Source: CAD feature listing. Evaluate the final solid. Frame: model axes, mm. Give positions to 0.01 mm unless a question says otherwise; leave off trailing zeros.
from build123d import *

# Parameters (mm, degrees)
SKETCH_1_R          = 3.2
SKETCH_1_R_2        = 2.5
EXTRUDE_1_DEPTH     = 3
SKETCH_2_R          = 2
SKETCH_2_R_2        = 1.75
CUT_EXTRUDE_1_DEPTH = 10


with BuildPart() as part:
    # Эскиз1 → Бобышка-Вытянуть1 (new body)
    with BuildSketch(Plane(origin=(0, 0, 0), x_dir=(1, 0, 0), z_dir=(0, 1, 0))):
        with BuildLine():
            Line((-65, -165), (65, -165))
            ThreePointArc((65, -165), (68.535533906, -163.535533906), (70, -160))
            Line((70, -160), (70, -120))
            ThreePointArc((70, -120), (72.928932188, -112.928932188), (80, -110))
            Line((80, -110), (192.5, -110))
            ThreePointArc((192.5, -110), (196.035533906, -108.535533906), (197.5, -105))
            Line((197.5, -105), (197.5, 105))
            ThreePointArc((197.5, 105), (196.035533906, 108.535533906), (192.5, 110))
            Line((192.5, 110), (80, 110))
            ThreePointArc((80, 110), (72.928932188, 112.928932188), (70, 120))
            Line((70, 120), (70, 160))
            ThreePointArc((70, 160), (68.535533906, 163.535533906), (65, 165))
            Line((65, 165), (-65, 165))
            ThreePointArc((-65, 165), (-68.535533906, 163.535533906), (-70, 160))
            Line((-70, 160), (-70, 120))
            ThreePointArc((-70, 120), (-72.928932188, 112.928932188), (-80, 110))
            Line((-80, 110), (-192.5, 110))
            ThreePointArc((-192.5, 110), (-196.035533906, 108.535533906), (-197.5, 105))
            Line((-197.5, 105), (-197.5, -105))
            ThreePointArc((-197.5, -105), (-196.035533906, -108.535533906), (-192.5, -110))
            Line((-192.5, -110), (-80, -110))
            ThreePointArc((-80, -110), (-72.928932188, -112.928932188), (-70, -120))
            Line((-70, -120), (-70, -160))
            ThreePointArc((-70, -160), (-68.535533906, -163.535533906), (-65, -165))
        make_face()
        with Locations((40, 146)):
            Circle(SKETCH_1_R, mode=Mode.SUBTRACT)
        with Locations((40, -146)):
            Circle(SKETCH_1_R, mode=Mode.SUBTRACT)
        with Locations((-40, -146)):
            Circle(SKETCH_1_R, mode=Mode.SUBTRACT)
        with Locations((-40, 146)):
            Circle(SKETCH_1_R, mode=Mode.SUBTRACT)
        with Locations((-178.768667216, 80)):
            Circle(SKETCH_1_R, mode=Mode.SUBTRACT)
        with Locations((-178.768667216, -80)):
            Circle(SKETCH_1_R, mode=Mode.SUBTRACT)
        with Locations((-178.768667216, 0)):
            Circle(SKETCH_1_R, mode=Mode.SUBTRACT)
        with Locations((178.768667216, 80)):
            Circle(SKETCH_1_R, mode=Mode.SUBTRACT)
        with Locations((178.768667216, 0)):
            Circle(SKETCH_1_R, mode=Mode.SUBTRACT)
        with Locations((178.768667216, -80)):
            Circle(SKETCH_1_R, mode=Mode.SUBTRACT)
        with Locations((137.5, -42)):
            Circle(SKETCH_1_R_2, mode=Mode.SUBTRACT)
        with Locations((159.5, -88)):
            Circle(SKETCH_1_R_2, mode=Mode.SUBTRACT)
        with Locations((115.5, -88)):
            Circle(SKETCH_1_R_2, mode=Mode.SUBTRACT)
        with Locations((-159.5, -88)):
            Circle(SKETCH_1_R_2, mode=Mode.SUBTRACT)
        with Locations((-137.5, -42)):
            Circle(SKETCH_1_R_2, mode=Mode.SUBTRACT)
        with Locations((-115.5, -88)):
            Circle(SKETCH_1_R_2, mode=Mode.SUBTRACT)
        with Locations((159.5, 88)):
            Circle(SKETCH_1_R_2, mode=Mode.SUBTRACT)
        with Locations((137.5, 42)):
            Circle(SKETCH_1_R_2, mode=Mode.SUBTRACT)
        with Locations((115.5, 88)):
            Circle(SKETCH_1_R_2, mode=Mode.SUBTRACT)
        with Locations((-115.5, 88)):
            Circle(SKETCH_1_R_2, mode=Mode.SUBTRACT)
        with Locations((-137.5, 42)):
            Circle(SKETCH_1_R_2, mode=Mode.SUBTRACT)
        with Locations((-159.5, 88)):
            Circle(SKETCH_1_R_2, mode=Mode.SUBTRACT)
    extrude(amount=EXTRUDE_1_DEPTH)

    # Эскиз2 → Вырез-Вытянуть1 (cut)
    with BuildSketch(Plane(origin=(0, 3, 0), x_dir=(1, 0, 0), z_dir=(0, 1, 0))):
        with Locations((128.5, 0)):
            Circle(SKETCH_2_R)
        with Locations((56.5, 0)):
            Circle(SKETCH_2_R)
        with Locations((93.5, 101)):
            Circle(SKETCH_2_R)
        with Locations((61.5, 54)):
            Circle(SKETCH_2_R)
        with Locations((53.5, 91.092247848)):
            Circle(SKETCH_2_R)
        with Locations((36.502982491, 78.046799413)):
            Circle(SKETCH_2_R)
        with Locations((28.680928288, 17.871923503)):
            Circle(SKETCH_2_R)
        with Locations((-27.319071712, 17.871923503)):
            Circle(SKETCH_2_R)
        with Locations((27.496289721, -46.022287392)):
            Circle(SKETCH_2_R_2)
        with Locations((93.5, -54.053341302)):
            Circle(SKETCH_2_R)
        with Locations((61.5, -101.042998556)):
            Circle(SKETCH_2_R)
        with Locations((53.5, -78.07249598)):
            Circle(SKETCH_2_R)
        with Locations((36.502982491, -90.999139468)):
            Circle(SKETCH_2_R)
        with Locations((27.496289721, -116.033195429)):
            Circle(SKETCH_2_R_2)
        with Locations((-27.552622159, -116.033195429)):
            Circle(SKETCH_2_R_2)
        with Locations((-27.319071712, -46)):
            Circle(SKETCH_2_R_2)
        with Locations((-53.636340651, -90.999139468)):
            Circle(SKETCH_2_R)
        with Locations((-36.401722668, -78.07249598)):
            Circle(SKETCH_2_R)
        with Locations((-93.526794479, -101.042998556)):
            Circle(SKETCH_2_R)
        with Locations((-61.727710595, -54.053341302)):
            Circle(SKETCH_2_R)
        with Locations((-36.401722668, 91.092247848)):
            Circle(SKETCH_2_R)
        with Locations((-53.636340651, 78.046799413)):
            Circle(SKETCH_2_R)
        with Locations((-61.541675198, 101)):
            Circle(SKETCH_2_R)
        with Locations((-93.526794479, 54)):
            Circle(SKETCH_2_R)
        with Locations((-128.5, 0)):
            Circle(SKETCH_2_R)
        with Locations((-56.5, 0)):
            Circle(SKETCH_2_R)
        with Locations((-16.832308482, 37.872518528)):
            Circle(SKETCH_2_R_2)
        with Locations((-16.797794126, 97.927570988)):
            Circle(SKETCH_2_R_2)
        with Locations((23.276008527, 97.927570988)):
            Circle(SKETCH_2_R_2)
        with Locations((23.276008527, 37.872518528)):
            Circle(SKETCH_2_R_2)
        with Locations((-0.75963633, 149.730797231)):
            Circle(SKETCH_2_R)
        with Locations((11.137406716, 149.864440097)):
            Circle(SKETCH_2_R)
        with Locations((11.137406716, 108.512875125)):
            Circle(SKETCH_2_R)
        with Locations((-0.627896327, 108.512875125)):
            Circle(SKETCH_2_R)
    extrude(amount=-CUT_EXTRUDE_1_DEPTH, mode=Mode.SUBTRACT)


solid = part.part
(1) Section A-A, the plane y = 2. Count the separate pieces of the cut face and the enclosed holes in it, plus the area to 3 significant figures.
(2) Line query: line 1 along Z through (x, y) = (61.5, 0.75); line 2 along X through (y, z) = (1.6, 88); line 3 along Z through (x, y) = (135.5, 1.5). Output: solid intervals per line, ascending.
(3) Pin query (flat end, axial travel): pin 1 Ø0.9 at (x, y) = (148, 2) entering from +Z. Return the tip coordinate at first contact, or that it passes through.
Checks:
1. separate pieces: 1
1. enclosed holes: 56
1. area: 101,000 mm2
2. line 1: z = -165 to -56, -52 to 99.04, 103.04 to 165
2. line 2: x = -197.5 to -162, -157 to -118, -113 to 113, 118 to 157, 162 to 197.5
2. line 3: z = -110 to -43.5, -40.5 to 40.5, 43.5 to 110
3. pin 1: stops at z = 110
